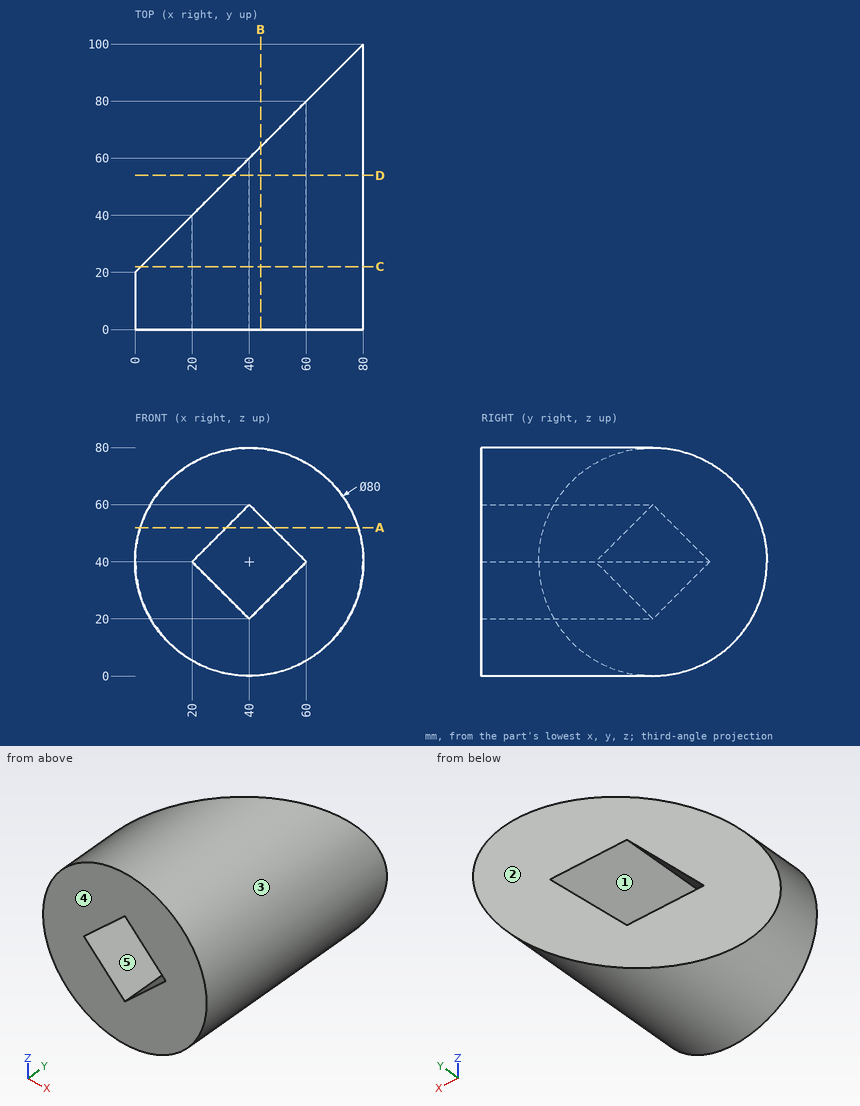
Drawing for the job (mm, zero at the part's lowest x, y, z). A direction names the side the tool comes from. Round coordinates to 2 decimals unless told otherwise and drop trailing zeros. Order: outer loops, then holes, each group sorted by start corner. A loop starts at its lowest first (then second) coordinate and runs counter-clockwise, first axis right, second up.
Item 1: Saw through at C-C on y = 22. Write the cut outline in (x, z), then the cut area to 3 significant figures.
Item 2: Tool access for the marked faces 4 and 5: list every direction of +Z, -Z, +X, -X, +Y, -Y with a clear straight run to the whole face (end or side of a thin tool).
Item 3: Saw through at D-D on y = 54. Write the cut outline in (x, z), then the cut area to 3 significant figures.
Item 4: Mould opens along X. For the marked faces 1, 2 and 3 say: pulls with the +X half, pulls with the -X half, needs draft (parallel to the pull), parting line crosses it, or undercut.
Item 5: Pin check, flat tips, straight feed: pin 1 (12 mm diameter, centred on y = 44, z = 69, fed in from -X); pin 2 (2 mm diameter, centred on x = 35.5, y = 35, fed in from -Z); pin 3 (5 mm diameter, centred on x = 15.5, z = 23, fed in from +Y). Stop position of each tip, or through.
Item 6: Saw through at B-B on x = 44. Write the cut outline in (y, z), then the cut area to 3 significant figures.
Item 7: Probe line 1 along Y through (x, z) = (20, 41.5); line 2 along Z through (x, y) = (46, 17); line 3 along Z through (x, y) = (53, 21). List the from-to ranges inside material, lowest first.
Item 8: Saw through at A-A on z = 52. Write the cut outline in (x, y).
Reported:
1. outline: (2, 27.51) arc R40 ccw (long way) to (2, 52.49) - close; hole (20, 40) - (40, 20) - (60, 40) - (40, 60) - close
1. area: 4,190 mm2
2. face 4: +Z, -Z, +X, -X, -Y
2. face 5: +Y, -Y
3. outline: (34, 0.45) arc R40 ccw (long way) to (34, 79.55) - (34, 54) - (40, 60) - (60, 40) - (40, 20) - (34, 26) - close
3. area: 2,390 mm2
4. face 1: undercut
4. face 2: pulls with the -X half
4. face 3: parting line crosses it
5. pin 1: stops at x = 18
5. pin 2: stops at z = 0.15
5. pin 3: stops at y = 38
6. outline: (0, 0.2) - (64, 0.2) - (64, 24) - (0, 24) - close; (0, 56) - (64, 56) - (64, 79.8) - (0, 79.8) - close
6. area: 3,050 mm2
7. line 1: y = 0 to 40
7. line 2: z = 0.45 to 26, 54 to 79.55
7. line 3: z = 2.17 to 33, 47 to 77.83
8. outline: (1.84, 0) - (32, 0) - (32, 52) - (1.84, 21.84) - close; (48, 0) - (78.16, 0) - (78.16, 98.16) - (48, 68) - close
